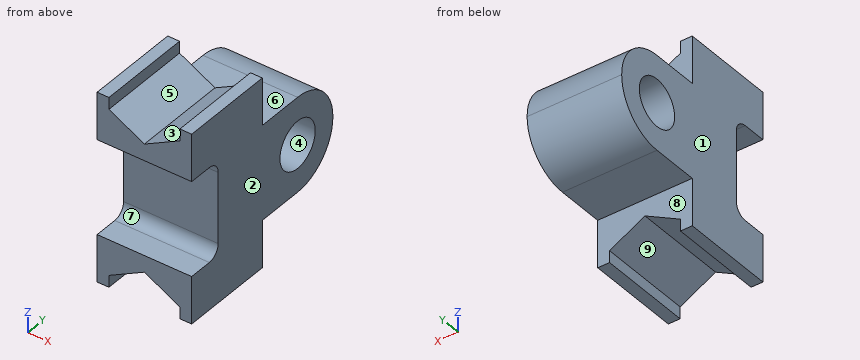
Autodesk Inventor part; units mm, degrees
ref_plane "YZ Plane" through (0, 0, 0) normal (1, 0, 0) x (0, 1, 0)
ref_plane "XZ Plane" through (0, 0, 0) normal (0, 1, 0) x (-1, 0, 0)
ref_plane "XY Plane" through (0, 0, 0) normal (0, 0, 1) x (1, 0, 0)
sketch "Esboço1" plane through (0, 0, 0) normal (0, 1, 0) x (-1, 0, 0)
  line L0 (20, 40) -> (-20, 40)
  line L1 (-20, 40) -> (-20, -40)
  line L2 (-20, -40) -> (20, -40)
  line L3 (20, -40) -> (20, 40)
  line L4 (20, 40) -> (-20, -40) construction
  line L5 (-20, 40) -> (20, -40) construction
  point P0 (0, 0)
  dimension "d0" = 40
  dimension "d1" = 80
extrude "Extrusão1" add sketch "Esboço1" along normal blind 80
sketch "Esboço2" plane through (20, 0, 40) normal (1, 0, 0) x (0, 0, -1)
  line L0 (0, 80) -> (80, 80)
  line L1 (0, 80) -> (20, 80)
  line L2 (20, 80) -> (20, 40)
  line L3 (20, 40) -> (0, 40)
  line L4 (0, 40) -> (0, 80)
  line L5 (80, 80) -> (60, 80)
  line L6 (60, 80) -> (60, 40)
  line L7 (60, 40) -> (80, 40)
  line L8 (80, 40) -> (80, 80)
  line L9 (0, 0) -> (80, 0)
  point P0 (40, 0)
  point P1 (60, 60)
  point P2 (20, 80)
  dimension "d4" = 40
  dimension "d5" = 20
  dimension "d6" = 20
extrude "Extrusão2" cut sketch "Esboço2" against normal blind 80
fillet "Arredondamento1" radius 20 2 edges at (0, 80, 20) (0, 80, -20)
sketch "Esboço3" plane through (20, 0, 40) normal (1, 0, 0) x (0, 0, -1)
  arc A0 (60, 60) -> (20, 60) centre (40, 60) ccw
  point P0 (40, 0)
hole "Furo1" at (20, 60, 0) direction (-1, 0, 0) diameter 20 end through all
sketch "Esboço4" plane through (20, 40, 40) normal (0, 1, 0) x (1, 0, 0)
  line L0 (0, 0) -> (0, 80)
  line L1 (0, 0) -> (-5, 0)
  line L2 (-40, 0) -> (0, 0)
  line L3 (-5, 0) -> (-5, 5)
  line L4 (-40, 0) -> (-35, 0)
  line L5 (-35, 0) -> (-35, 5)
  line L6 (-35, 0) -> (-20, 0) construction
  line L7 (-20, 0) -> (-20, 13) construction
  line L8 (-35, 5) -> (-20, 13)
  line L9 (-20, 13) -> (-5, 5)
  point P0 (-20, 40)
  dimension "d17" = 5
  dimension "d18" = 5
  dimension "d19" = 5
  dimension "d20" = 15
  dimension "d21" = 13
extrude "Extrusão3" cut sketch "Esboço4" against normal blind 80
mirror "Espelhar1" about plane through (0, 0, 0) normal (0, 0, 1) of "Extrusão3"
sketch "Esboço5" plane through (20, 0, 40) normal (1, 0, 0) x (0, 0, -1)
  point P0 (40, 0)
sketch "Esboço6" plane through (20, 0, 40) normal (1, 0, 0) x (0, 0, -1)
  line L0 (0, 0) -> (0, 40) construction
  line L1 (0, 0) -> (20, 0) construction
  line L2 (0, 0) -> (80, 0) construction
  line L3 (20, 0) -> (20, 15)
  line L4 (20, 15) -> (60, 15)
  line L5 (60, 15) -> (60, 0)
  line L6 (60, 0) -> (20, 0)
  point P0 (40, 0)
  dimension "d24" = 20
  dimension "d25" = 15
  dimension "d26" = 40
extrude "Extrusão4" cut sketch "Esboço6" against normal blind 80
fillet "Arredondamento2" radius 5 2 edges at (0, 15, -20) (0, 15, 20)
Verification items for the finished model (mm, model axes). Face numbers are marked on the shaded views. A direction names the side the tool comes from. Coordinates: 2 decimals unless noted, no trailing zeros. Order: outer loops, then holes, each group sorted by start corner. A loop starts at its lowest first (then second) coordinate and runs counter-clockwise, first axis right, second up.
Item 1: Depth check by flat-ended pin: pin 1 (12 mm diameter, centred on y = 60, z = 0, fed in from -X); pin 2 (16 mm diameter, centred on x = 7.5, z = 26.5, fed in from +Y); pin 3 (4 mm diameter, centred on x = -9, y = 54, fed in from +Z); pin 4 (6 mm diameter, centred on x = 6.5, y = 34, fed in from -Z). Enter the tip coordinate at first touch or a pass-through.
Filled in:
pin 1: passes through
pin 2: stops at y = 67.6
pin 3: stops at z = 20
pin 4: stops at z = -32.07
Item 2: Release check for a two-part mould opening along X. For the marked faces 1, 2, 3 and 4 record: +X half, -X half, draft (parallel to the pull), parting line (faces both ways), or undercut.
Filled in:
face 1: -X half
face 2: +X half
face 3: undercut
face 4: draft
Item 3: Section check B-B, the plane y = 56. Enter the section's corners in (x, z).
Filled in:
outline: (-20, -20) - (20, -20) - (20, -9.17) - (-20, -9.17) - close; (-20, 9.17) - (20, 9.17) - (20, 20) - (-20, 20) - close
Item 4: Access from +Z, -Z, +X, -X, +Y, -Y to the whole of each face (thin tool, end or side, straight path). Record for the marked faces 5, 6, 7, 8 and 9.
Filled in:
face 5: +Z, +Y, -Y
face 6: +Z, +X, -X, +Y
face 7: +X, -X, -Y
face 8: -Z, +X, -X, +Y
face 9: -Z, +Y, -Y
Item 5: Material ranges on L1, parallel to Y at x = -7, z = 0; L2, parallel to Z at x = 1, y = 60; L3, parallel to X at y = 27, z = 36.5, recorded low to high.
Filled in:
L1: y = 15 to 50, 70 to 80
L2: z = -20 to -10, 10 to 20
L3: x = -20 to -15, 15 to 20
Item 6: Section check D-D, the plane y = 44.5. Enter the section's corners in (x, z).
Filled in:
outline: (-20, -20) - (20, -20) - (20, 20) - (-20, 20) - close
Item 7: Section check A-A, the plane z = 29. Enter the section's corners in (x, y), then the cut area to 3 significant figures.
Filled in:
outline: (-20, 0) - (-3.75, 0) - (-3.75, 40) - (-20, 40) - close; (3.75, 0) - (20, 0) - (20, 40) - (3.75, 40) - close
area: 1,300 mm2
